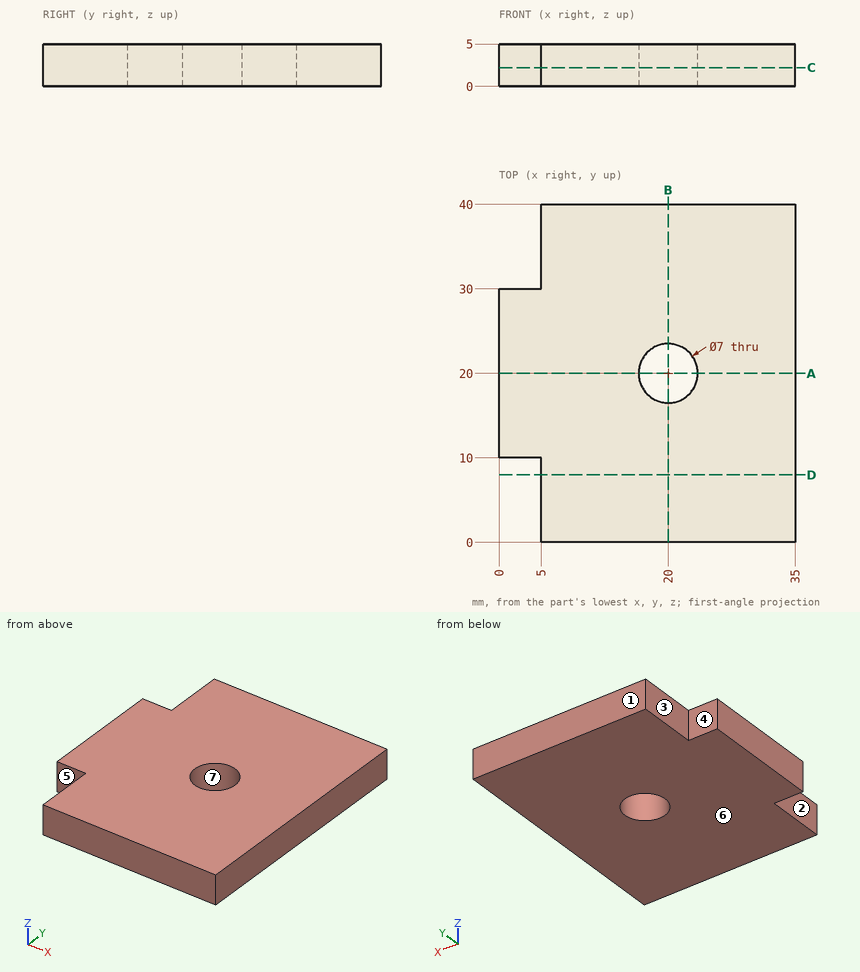
Could you check a few things on this drawing? It's one solid part, dimensions in mm from its lowest x, y, z. A direction names the side the tool comes from. Coordinates: 2 decimals unless noted, no trailing zeros. Loops run counter-clockwise (first coordinate to the right, second up) from the corner with the lowest first, then second, coordinate; pieces in that order, holes last. Notation, with made-up numbers: (18, 70) - (49, 70) arc R15 ccw to (49, 88) - close; hole circle Ø4 at (17.5, 33.5). An arc over 180 degrees is marked (long way). Answer as a JSON object with one key per item and string values. Group by question number.
Item 1: If we section it at A-A (y = 20): List the corners of the cut face in (x, z) for me, plus the area to 3 significant figures.
Item 2: If we mould it in two halves opening along Y, with no side actions, what happens to the marked faces 4, 5, 6 and 7? For each: released by +Y, released by -Y, zero draft, split by the parting line, or undercut.
Item 3: For pin 1 (2.5 mm diameter, centred on x = 2, z = 1.5, fed in from -Y); pin 2 (8 mm diameter, centred on x = 10.5, y = 12, fed in from -Z); pin 3 (6.5 mm diameter, centred on x = 20, y = 20, fed in from +Z), each with a flat end and sliding along its axis, tell me the tip position at first contact or that it passes through.
Item 4: If we section it at D-D (y = 8): List the corners of the cut face in (x, z) for me.
Item 5: If we section it at C-C (z = 2.2): List the corners of the cut face in (x, y) for me, plus the area to 3 significant figures.
Item 6: If we section it at B-B (x = 20): List the corners of the cut face in (y, z) for me, plus the area to 3 significant figures.
Item 7: On a 3-axis mill with a long thin cutter (end or side, diameter ignored), from which of +Z, -Z, +X, -X, +Y, -Y can I reach the whole of each face in a straight line? I mean the marked faces 1, 2 and 3. Say none if no direction works.
Item 8: If I drill on L1, parallel to Y at x = 20, z = 1.8; L2, parallel to X at y = 5.5, z = 3.85; L3, parallel to X at y = 18.5, z = 2.2, over which ranges is the centre line in solid material (lowest first)? Write a range as from..to.
Returned:
{
 "1": {"outline": "(0, 0) - (16.5, 0) - (16.5, 5) - (0, 5) - close; (23.5, 0) - (35, 0) - (35, 5) - (23.5, 5) - close", "area": "140 mm²"},
 "2": {"face 4": "released by +Y", "face 5": "released by -Y", "face 6": "zero draft", "face 7": "undercut"},
 "3": {"pin 1": "stops at y = 10", "pin 2": "stops at z = 0", "pin 3": "passes through"},
 "4": {"outline": "(5, 0) - (35, 0) - (35, 5) - (5, 5) - close"},
 "5": {"outline": "(0, 10) - (5, 10) - (5, 0) - (35, 0) - (35, 40) - (5, 40) - (5, 30) - (0, 30) - close; hole circle Ø7 at (20, 20)", "area": "1,260 mm²"},
 "6": {"outline": "(0, 0) - (16.5, 0) - (16.5, 5) - (0, 5) - close; (23.5, 0) - (40, 0) - (40, 5) - (23.5, 5) - close", "area": "165 mm²"},
 "7": {"face 1": "+Z, -Z, +X, -X, +Y", "face 2": "+Z, -Z, -X, -Y", "face 3": "+Z, -Z, -X, +Y"},
 "8": {"L1": "y = 0..16.5, 23.5..40", "L2": "x = 5..35", "L3": "x = 0..16.84, 23.16..35"}
}
